```python
from build123d import *

# Parameters (mm, degrees)
SKETCH_1_R          = 9.52
EXTRUDE_1_DEPTH     = 4
SKETCH_4_W          = 46.2
SKETCH_4_H          = 8.602857229
EXTRUDE_2_DEPTH     = 4
SKETCH_2_R          = 2
SKETCH_2_R_2        = 1.5
SKETCH_2_W          = 8.2
SKETCH_2_H          = 4.2
CUT_EXTRUDE_1_DEPTH = 4
CUT_EXTRUDE_2_DEPTH = 10
FILLET_1_R          = 2


with BuildPart() as part:
    # 草图1 → 凸台-拉伸1 (new body)
    with BuildSketch(Plane.XY):
        with BuildLine():
            Line((328.542857143, -40.145714286), (-1.457142857, -40.145714286))
            ThreePointArc((-1.457142857, -40.145714286), (-41.457142857, -0.145714286), (-1.457142857, 39.854285714))
            Line((-1.457142857, 39.854285714), (328.542857143, 39.854285714))
            ThreePointArc((328.542857143, 39.854285714), (368.542857143, -0.145714286), (328.542857143, -40.145714286))
        make_face()
        with Locations((-1.457142857, -0.145714286)):
            Circle(SKETCH_1_R, mode=Mode.SUBTRACT)
        with Locations((328.542857143, -0.145714286)):
            Circle(SKETCH_1_R, mode=Mode.SUBTRACT)
    extrude(amount=EXTRUDE_1_DEPTH)

    # 草图4 → 凸台-拉伸2 (add)
    with BuildSketch(Plane.XY.offset(4)):
        with Locations((18.542857143, 39.652857099)):
            Rectangle(SKETCH_4_W, SKETCH_4_H)
    extrude(amount=-EXTRUDE_2_DEPTH)

    # 草图2 → 切除-拉伸1 (cut)
    with BuildSketch(Plane.XY.offset(4)):
        with Locations((108.542857143, 33.854285714)):
            Circle(SKETCH_2_R)
        with Locations((198.542857143, 33.854285714)):
            Circle(SKETCH_2_R)
        with Locations((288.542857143, 33.854285714)):
            Circle(SKETCH_2_R)
        with Locations((108.542857143, -34.145714286)):
            Circle(SKETCH_2_R)
        with Locations((198.542857143, -34.145714286)):
            Circle(SKETCH_2_R)
        with Locations((288.542857143, -34.145714286)):
            Circle(SKETCH_2_R)
        with Locations((18.542857143, -34.145714286)):
            Circle(SKETCH_2_R)
        with Locations((18.542857143, 40.014285714)):
            Circle(SKETCH_2_R_2)
        Polygon((31.542857143, -21.145714286), (104.183898028, -21.145714286), (159.772133322, 20.854285714), (31.542857143, 20.854285714), align=None)
        Polygon((275.542857143, 20.854285714), (202.901816258, 20.854285714), (147.313580964, -21.145714286), (275.542857143, -21.145714286), align=None)
        with Locations((33.542857143, 40.014285714)):
            Rectangle(SKETCH_2_W, SKETCH_2_H)
        with Locations((3.542857143, 40.014285714)):
            Rectangle(SKETCH_2_W, SKETCH_2_H)
    extrude(amount=-CUT_EXTRUDE_1_DEPTH, mode=Mode.SUBTRACT)

    # 草图3 → 切除-拉伸2 (cut)
    with BuildSketch(Plane.XY.offset(4)):
        with BuildLine():
            Line((183.145474057, 18.460683743), (155.35135641, -2.539316257))
            ThreePointArc((155.35135641, -2.539316257), (151.149255171, -1.954213553), (151.734357875, 2.247887686))
            Line((151.734357875, 2.247887686), (179.528475522, 23.247887686))
            ThreePointArc((179.528475522, 23.247887686), (183.730576762, 22.662784982), (183.145474057, 18.460683743))
        make_face()
    extrude(amount=-CUT_EXTRUDE_2_DEPTH, mode=Mode.SUBTRACT)

    # 圆角1
    fillet_1_edges = [part.edges().sort_by_distance(p)[0] for p in [
        (31.542857143, -21.145714286, 2),
        (31.542857143, 20.854285714, 2),
        (159.772133322, 20.854285714, 2),
        (104.183898028, -21.145714286, 2),
        (275.542857143, 20.854285714, 2),
        (275.542857143, -21.145714286, 2),
        (147.313580964, -21.145714286, 2),
        (202.901816258, 20.854285714, 2),
    ]]
    fillet(fillet_1_edges, radius=FILLET_1_R)


solid = part.part
```
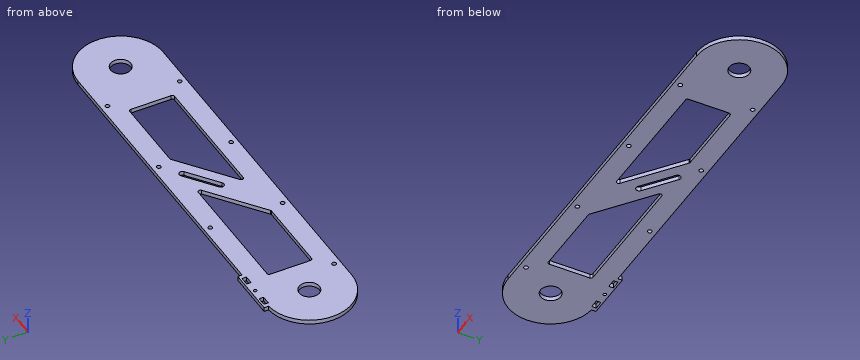
The listing builds one solid part. Answer for the finished solid, in the listing's coordinates (mm). Round coordinates to 2 decimals unless told otherwise and drop trailing zeros. Write each loop counter-clockwise with the first axis right and the second up, starting at its lowest first coordinate (ties: lowest second). Pieces come first, ordered by that corner, then holes. Notation, with made-up numbers: (-13.75, 42) -> (40.25, 42) arc R25 ccw to (40.25, 66) -> close; hole circle Ø11 at (56.25, -31.5). An arc over 180 degrees is marked (long way). Use CSV: the item, a comma, the result in double quotes. Start each with the question number.
(1) Each of these flat-tipped pins is pushed along its axis until it touches: pin 1 (1.2 mm diameter, centred on y = -6, z = 2, fed in from -X); pin 2 (2 mm diameter, centred on y = 6.5, z = 1.5, fed in from +X); pin 3 (2 mm diameter, centred on x = 161.5, z = 1.5, fed in from +Y). Where does it stop, or does it pass through?
(2) Section A-A on x = 269.5 is taken. Give the vertices of the cut face in (y, z), then the cut area to 3 significant figures.
(3) Consider L1, parallel to Y at x = 44.5, z = 1.6; L2, parallel to X at y = 12, z = 2.1; L3, parallel to X at y = 1, z = 2.3. Determine where each line is inside the solid, lowest interval first. Write a range as from..to.
(4) Section D-D on z = 2.25 is taken. Count the separate pieces of the cut face and the enclosed holes in it, then the cut area to 3 significant figures.
(5) Section B-B on x = 121 is taken. Give the vertices of the cut face in (y, z), then the cut area to 3 significant figures.
(6) Section C-C on y = -27 is taken. Give the vertices of the cut face in (x, z).
A:
1,pin 1,"stops at x = -41.11"
1,pin 2,"stops at x = 368.14"
1,pin 3,"stops at y = 39.85"
2,outline,"(-40.15, 0) -> (-21.15, 0) -> (-21.15, 4) -> (-40.15, 4) -> close; (20.85, 0) -> (39.85, 0) -> (39.85, 4) -> (20.85, 4) -> close"
2,area,"152 mm²"
3,L1,"y = -40.15..-21.15, 20.85..39.85"
3,L2,"x = -39.57..31.54, 148.05..164.64, 174.59..191.18, 275.54..366.65"
3,L3,"x = -41.44..-10.91, 7.99..31.54, 133.49..150.77, 160.04..176.62, 275.54..319.09, 337.99..368.53"
4,separate pieces,"1"
4,enclosed holes,"15"
4,area,"22,200 mm²"
5,outline,"(-40.15, 0) -> (-8.44, 0) -> (-8.44, 4) -> (-40.15, 4) -> close; (20.85, 0) -> (39.85, 0) -> (39.85, 4) -> (20.85, 4) -> close"
5,area,"203 mm²"
6,outline,"(-31.1, 0) -> (358.19, 0) -> (358.19, 4) -> (-31.1, 4) -> close"
